Verification items for the finished model (mm, model axes). Coordinates: 2 decimals unless noted, no trailing zeros. Loops run counter-clockwise (first coordinate to the right, second up) from the corner with the lowest first, then second, coordinate; pieces in that order, holes last. Notation, with made-up numbers: (-38.5, 15) -> (-4.5, 15) arc R16 ccw to (-4.5, 32) -> close; hole circle Ø11 at (-33.5, -17.5). An arc over 180 degrees is marked (long way). Answer as a JSON object with one key per item and string values. Group by question number.
Q1. Gauge pin test, flat ends, axial feed: pin 1 Ø3 at (x, z) = (7, -2) entering from +Y; pin 2 Ø0.7 at (y, z) = (-3, -5) entering from -X; pin 3 Ø6 at (y, z) = (3, 4.5) entering from +X. Record the tip position at first contact, or that the pin passes through.
Q2. Cross-section at A-A on x = 2.5. Record the boundary of the cut face in (y, z).
Q3. Release check for a two-part mould opening along Y. For faces 1 (the flat face through (0, 1.6, -3.4)), 2 (the flat face through (1, -3.552, 0)), 3 (the flat face through (2.1, -3, 5)), 4 (the cylindrical face through (2.218, -0.33, -7.493)) record: released by +Y, released by -Y, zero draft, split by the parting line, or undercut.
Q4. Cross-section at D-D on y = 5.5. Record the boundary of the cut face in (x, z), and give its area (3 significant figures).
Q5. Scan lines: L1, parallel to Y at x = 1.2, z = 0; L2, parallel to Y at x = 1.75, z = 1.5; L3, parallel to Z at x = 2.5, y = -1. Record each from-to range of solid material in increasing order.
Q6. Cross-section at C-C on y = 2. Record the boundary of the cut face in (x, z), and give its area (3 significant figures).
Q7. Cross-section at B-B on z = 0. Record the boundary of the cut face in (x, y).
```python
from build123d import *

# Parameters (mm, degrees)
CUT_EXTRUDE1_DEPTH = 2.75
SKETCH3_R          = 1.127
CUT_EXTRUDE2_DEPTH = 2.1


with BuildPart() as part:
    # Sketch1 → Revolve1 (revolve)
    with BuildSketch(Plane.XY, mode=Mode.PRIVATE) as revolve1_sk:
        with BuildLine():
            Line((0, 0), (12, 0))
            ThreePointArc((12, 0), (9.803300859, -5.303300859), (4.5, -7.5))
            Line((4.5, -7.5), (0, -7.5))
            Line((0, -7.5), (0, 0))
        make_face()
    revolve(revolve1_sk.sketch.rotate(Axis((0, 0, 0), (1, 0, 0)), 270), axis=Axis((0, 0, 0), (1, 0, 0)))

    # Sketch2 → Cut-Extrude1 (cut)
    with BuildSketch(Plane.ZY):
        Polygon((2.050748156, 3.552), (-2.050748156, 3.552), (-4.101496312, 0), (-2.050748156, -3.552), (2.050748156, -3.552), (4.101496312, 0), align=None)
    extrude(amount=-CUT_EXTRUDE1_DEPTH, mode=Mode.SUBTRACT)

    # Sketch3 → Cut-Extrude2 (cut)
    with BuildSketch(Plane.ZY):
        with Locations((-4.763139721, -2.75)):
            Circle(SKETCH3_R)
        with Locations((0, 5.5)):
            Circle(SKETCH3_R)
        with Locations((4.763139721, -2.75)):
            Circle(SKETCH3_R)
    extrude(amount=-CUT_EXTRUDE2_DEPTH, mode=Mode.SUBTRACT)


solid = part.part
```
Computed values:
{
 "1": {"pin 1": "stops at y = 7.3", "pin 2": "stops at x = 2.1", "pin 3": "stops at x = 11.6"},
 "2": {"outline": "circle Ø15 at (0, 0); hole (-3.55, -2.05) -> (0, -4.1) -> (3.55, -2.05) -> (3.55, 2.05) -> (0, 4.1) -> (-3.55, 2.05) -> close"},
 "3": {"face 1": "zero draft", "face 2": "undercut", "face 3": "undercut", "face 4": "split by the parting line"},
 "4": {"outline": "(0, -5.1) -> (4.5, -5.1) arc R5.1 ccw to (4.5, 5.1) -> (0, 5.1) -> (0, 1.13) -> (2.1, 1.13) -> (2.1, -1.13) -> (0, -1.13) -> close", "area": "82.0 mm²"},
 "5": {"L1": "y = -7.5 to -3.55, 3.55 to 4.37, 6.63 to 7.5", "L2": "y = -7.35 to -3.55, 3.55 to 7.35", "L3": "z = -7.43 to -3.52, 3.52 to 7.43"},
 "6": {"outline": "(0, -7.23) -> (4.5, -7.23) arc R7.23 ccw to (4.5, 7.23) -> (0, 7.23) -> (0, 2.95) -> (2.75, 2.95) -> (2.75, -2.95) -> (0, -2.95) -> close", "area": "131 mm²"},
 "7": {"outline": "(0, -7.5) -> (4.5, -7.5) arc R7.5 ccw to (4.5, 7.5) -> (0, 7.5) -> (0, 6.63) -> (2.1, 6.63) -> (2.1, 4.37) -> (0, 4.37) -> (0, 3.55) -> (2.75, 3.55) -> (2.75, -3.55) -> (0, -3.55) -> close"}
}
